from build123d import *

# Parameters (mm, degrees)
AUFSATZ_LINEAR_AUSTRAGEN1_DEPTH = 3
DURCHGANGSLOCH_F_R_M51_D        = 5.5
VERRUNDUNG1_R                   = 2


with BuildPart() as part:
    # Skizze1 → Aufsatz-Linear austragen1 (new body)
    with BuildSketch(Plane.XY):
        Polygon((0, 0), (0, 47), (-18, 47), (-18, -18), (47, -18), (47, 0), align=None)
    extrude(amount=AUFSATZ_LINEAR_AUSTRAGEN1_DEPTH)

    # Durchgangsloch für M51 (through all)
    with Locations(Plane.XY.offset(3)):
        with Locations((17, -9), (-9, 37), (-9, 17), (37, -9)):
            Hole(DURCHGANGSLOCH_F_R_M51_D / 2)

    # Verrundung1
    verrundung1_edges = [part.edges().sort_by_distance(p)[0] for p in [
        (47, 0, 1.5),
        (47, -18, 1.5),
        (-18, -18, 1.5),
        (-18, 47, 1.5),
        (0, 47, 1.5),
    ]]
    fillet(verrundung1_edges, radius=VERRUNDUNG1_R)


solid = part.part
Read the model definition and answer for the solid it produces. Units are mm, in the model's axes. A direction names the side the tool comes from. Round coordinates to 2 decimals unless told otherwise and drop trailing zeros. Write each loop counter-clockwise with the first axis right and the second up, starting at its lowest first coordinate (ties: lowest second). Pieces come first, ordered by that corner, then holes. Notation, with made-up numbers: M 6,57.25 L 17,57.25 A20 cw 17,70.25 Z; hole C 33,41 d8. An arc over 180 degrees is marked long. Use a Markdown table: item, result.
1) A tool of negligible diameter and unlimited length cuts with its end or side. For faces 1 (the cylindrical face through (-17.43, -17.4, 1.52)), 2 (the flat face through (23, 0, 1)), from which of +Z, -Z, +X, -X, +Y, -Y can it reach the whole face along a straight path? Write none if from no direction.
Answers follow:
| item | result |
|---|---|
| face 1 | +Z, -Z, -X, -Y |
| face 2 | +Z, -Z, +X, +Y |
2) Straight lines are drawn through the part: line 1 along Y through (x, z) = (-9, 1.75); line 2 along Y through (x, z) = (17, 1.35); line 3 along Y through (x, z) = (7, 1.55). For each, find the intervals that lie inside material, in ascending order. Write a range as [from, to].
Answers follow:
| item | result |
|---|---|
| line 1 | y = [-18, 14.25], [19.75, 34.25], [39.75, 47] |
| line 2 | y = [-18, -11.75], [-6.25, 0] |
| line 3 | y = [-18, 0] |
3) A flat-ended cylindrical pin translates along its axis: pin 1 (5 mm diameter, centred on x = -9, y = 17, fed in from +Z). Find the tip coordinate at first contact, or state that the pin passes through.
Answers follow:
| item | result |
|---|---|
| pin 1 | passes through |
4) The part is cut by section D-D (z = 1.1). Write down the section's boundary in (x, y).
Answers follow:
| item | result |
|---|---|
| outline | M -18,-16 A2 ccw -16,-18 L 45,-18 A2 ccw 47,-16 L 47,-2 A2 ccw 45,0 L 0,0 L 0,45 A2 ccw -2,47 L -16,47 A2 ccw -18,45 Z; hole C -9,17 d5.5; hole C -9,37 d5.5; hole C 17,-9 d5.5; hole C 37,-9 d5.5 |
5) The part is cut by section A-A (x = -9). Write down the section's boundary in (y, z), plus the area to 3 significant figures.
Answers follow:
| item | result |
|---|---|
| outline | M -18,0 L 14.25,0 L 14.25,3 L -18,3 Z; M 19.75,0 L 34.25,0 L 34.25,3 L 19.75,3 Z; M 39.75,0 L 47,0 L 47,3 L 39.75,3 Z |
| area | 162 mm2 |
6) The part is cut by section B-B (y = 17). Write down the section's boundary in (x, z).
Answers follow:
| item | result |
|---|---|
| outline | M -18,0 L -11.75,0 L -11.75,3 L -18,3 Z; M -6.25,0 L 0,0 L 0,3 L -6.25,3 Z |
7) For a pull along X with two mould halves and no side action, classify faces 3 (the flat face through (0, 22, 1)), 4 (the cylindrical face through (-8.642, 19.727, 1.479)), 5 (the cylindrical face through (-17.4, 46.43, 1.52)), 6 (the flat face through (-0.4, 7.7, 0)) as pulls with the +X half, pulls with the -X half, needs draft (parallel to the pull), parting line crosses it, or undercut.
Answers follow:
| item | result |
|---|---|
| face 3 | pulls with the +X half |
| face 4 | undercut |
| face 5 | pulls with the -X half |
| face 6 | needs draft |
